Input: dimensioned drawing with shaded views. Units: mm. Origin: part minimum x, y, z. A direction names the side the tool comes from. Round coordinates to 2 decimals unless told otherwise and drop trailing zeros. Loops run counter-clockwise (first coordinate to the right, second up) from the corner with the lowest first, then second, coordinate; pieces in that order, holes last. Notation, with made-up numbers: (57, 4) - (116, 4) arc R16 cw to (116, 24) - close; hole circle Ø1 at (14.5, 22). An arc over 180 degrees is marked (long way). Answer as a JSON object with one key per item and string values. Group by question number.
Item 1: First-contact query: pin 1 (2 mm diameter, centred on y = 8, z = 11.5, fed in from +X); pin 2 (12.5 mm diameter, centred on y = 9.5, z = 14.5, fed in from -X); pin 3 (2 mm diameter, centred on y = 39.5, z = 19, fed in from -X). Flat tips, straight axial feed; report the tip coordinate or a pass-through.
Item 2: Reachability of the marked faces 1, 2 and 3 from +Z, -Z, +X, -X, +Y, -Y: full face, straight path, thin tool, end or side. Return the list, or none.
Item 3: Draft query along X for the marked faces 4, 5, 6 and 7. Return one class per face: released by +X, released by -X, zero draft, split by the parting line, or undercut.
Item 4: Section C-C (z = 16.5). Return the cut outline in (x, y), plus the area to 3 significant figures.
Item 5: Line query: line 1 (X direction, y = 3, z = 23.5); line 2 (Y direction, x = 6, z = 26); line 3 (X direction, y = 15.5, z = 12.5). Output: solid intervals per line, ascending.
Item 6: Section B-B (x = 14). Return the cut outline in (y, z), plus the area to 3 significant figures.
Item 7: Section A-A (y = 5). Return the cut outline in (x, z), plus the area to 3 significant figures.
Item 8: Section D-D (y = 13). Return the cut outline in (x, z), plus the area to 3 significant figures.
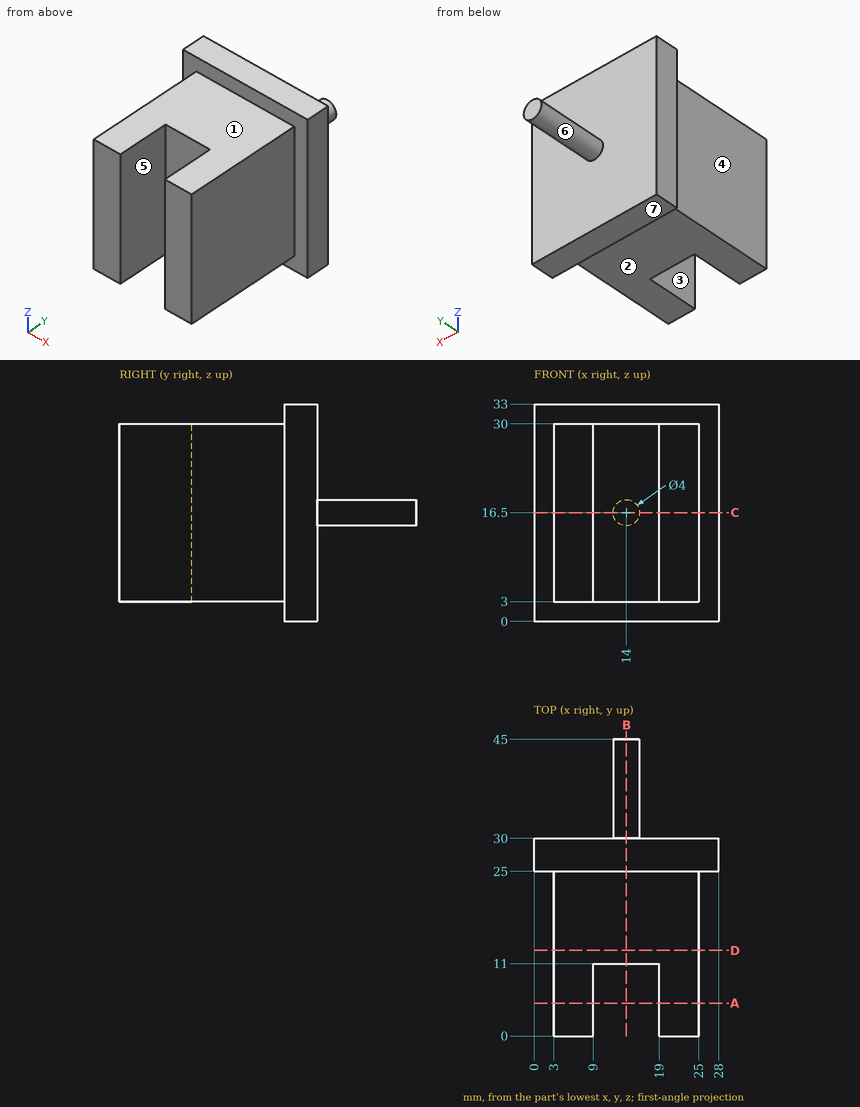
Values:
{
 "1": {"pin 1": "stops at x = 25", "pin 2": "stops at x = 3", "pin 3": "stops at x = 12.68"},
 "2": {"face 1": "+Z, +X, -X, -Y", "face 2": "-Z, +X, -X, -Y", "face 3": "+Z, -Z, -Y"},
 "3": {"face 4": "released by -X", "face 5": "undercut", "face 6": "split by the parting line", "face 7": "zero draft"},
 "4": {"outline": "(0, 25) - (3, 25) - (3, 0) - (9, 0) - (9, 11) - (19, 11) - (19, 0) - (25, 0) - (25, 25) - (28, 25) - (28, 30) - (16, 30) - (16, 45) - (12, 45) - (12, 30) - (0, 30) - close", "area": "640 mm^2"},
 "5": {"line 1": "x = 3 to 9, 19 to 25", "line 2": "y = 0 to 30", "line 3": "x = 3 to 25"},
 "6": {"outline": "(11, 3) - (25, 3) - (25, 0) - (30, 0) - (30, 14.5) - (45, 14.5) - (45, 18.5) - (30, 18.5) - (30, 33) - (25, 33) - (25, 30) - (11, 30) - close", "area": "603 mm^2"},
 "7": {"outline": "(3, 3) - (9, 3) - (9, 30) - (3, 30) - close; (19, 3) - (25, 3) - (25, 30) - (19, 30) - close", "area": "324 mm^2"},
 "8": {"outline": "(3, 3) - (25, 3) - (25, 30) - (3, 30) - close", "area": "594 mm^2"}
}
